Input: part model. Units: mm. Frame: model coordinates. Face numbers are marked on the shaded views. Coordinates: 2 decimals unless noted, no trailing zeros. Write each loop counter-clockwise with the first axis right and the second up, starting at its lowest first coordinate (ties: lowest second). Pieces come first, ordered by that corner, then holes.
1) Section query D-D (x = 42.5). Output: boundary loops of the cut face in (y, z), then the cut area to 3 significant figures.
2) Pin query (flat end, axial travel): pin 1 Ø4 at (x, y) = (44.5, 4) entering from +Z; pin 2 Ø5 at (x, z) = (67, -22) entering from +Y; pin 3 Ø16 at (x, z) = (38.09, -19.05) entering from +Y. Return the tip coordinate at first contact, or that it passes through.
3) Draft query along X for the marked faces 1, 2, 3 and 4. Return one class per face: pulls with the +X half, pulls with the -X half, needs draft (parallel to the pull), parting line crosses it, or undercut.
4) Section query B-B (y = 15). Output: boundary loops of the cut face in (x, z) (3 decimals), then the cut area to 3 significant figures.
5) Line query: L1, parallel to X at y = 8, z = -12.5; L2, parallel to Y at x = 38, z = -1.5; L3, parallel to X at y = 1.5, z = -19.05. Output: solid intervals per line, ascending.
6) Section query A-A (z = -19.05). Output: boundary loops of the cut face in (x, y), then the cut area to 3 significant figures.
7) Section query C-C (z = -3.5). Output: boundary loops of the cut face in (x, y), then the cut area to 3 significant figures.
from build123d import *

# Parameters (mm, degrees)
SKETCH1_W           = 76.2
SKETCH1_H           = 38.1
BOSS_EXTRUDE1_DEPTH = 25.4
SKETCH2_R           = 11.43
CUT_EXTRUDE1_DEPTH  = 89.9
SKETCH5_W           = 25.4
SKETCH5_H           = 5.08
CUT_EXTRUDE3_DEPTH  = 89.890839867
SKETCH3_R           = 3.302
CUT_EXTRUDE6_DEPTH  = 89.890839867
CUT_EXTRUDE7_START  = -7.62
SKETCH3_3_R         = 6.985
SKETCH3_3_R_2       = 3.302
CUT_EXTRUDE7_DEPTH  = 10.16


with BuildPart() as part:
    # Sketch1 → Boss-Extrude1 (new body)
    with BuildSketch(Plane(origin=(0, 0, 0), x_dir=(1, 0, 0), z_dir=(0, 1, 0))):
        with Locations((38.089312979, 19.05)):
            Rectangle(SKETCH1_W, SKETCH1_H)
    extrude(amount=BOSS_EXTRUDE1_DEPTH)

    # Sketch2 → Cut-Extrude1 (cut, through all)
    with BuildSketch(Plane.ZY.offset(0.010687021)):
        with Locations((-19.05, 25.4)):
            Circle(SKETCH2_R)
    extrude(amount=-CUT_EXTRUDE1_DEPTH, mode=Mode.SUBTRACT)

    # Sketch5 → Cut-Extrude3 (cut, through all)
    with BuildSketch(Plane(origin=(0, 0, -38.1), x_dir=(-1, 0, 0), z_dir=(0, 0, -1))):
        with Locations((-35.549312979, 8.89)):
            Rectangle(SKETCH5_W, SKETCH5_H)
    extrude(amount=-CUT_EXTRUDE3_DEPTH, mode=Mode.SUBTRACT)

    # Sketch3 → Cut-Extrude6 (cut, through all)
    with BuildSketch(Plane.XZ):
        with Locations(Location((38.089312979, -19.05, 0), (0, 0, 270))):
            Circle(SKETCH3_R)
    extrude(amount=-CUT_EXTRUDE6_DEPTH, mode=Mode.SUBTRACT)

    # Sketch3_3 → Cut-Extrude7 (cut)
    with BuildSketch(Plane.XZ.offset(CUT_EXTRUDE7_START)):
        with Locations(Location((38.089312979, -19.05, 0), (0, 0, 90))):
            Circle(SKETCH3_3_R)
        with Locations(Location((38.089312979, -19.05, 0), (0, 0, 270))):
            Circle(SKETCH3_3_R_2, mode=Mode.SUBTRACT)
    extrude(amount=-CUT_EXTRUDE7_DEPTH, mode=Mode.SUBTRACT)


solid = part.part
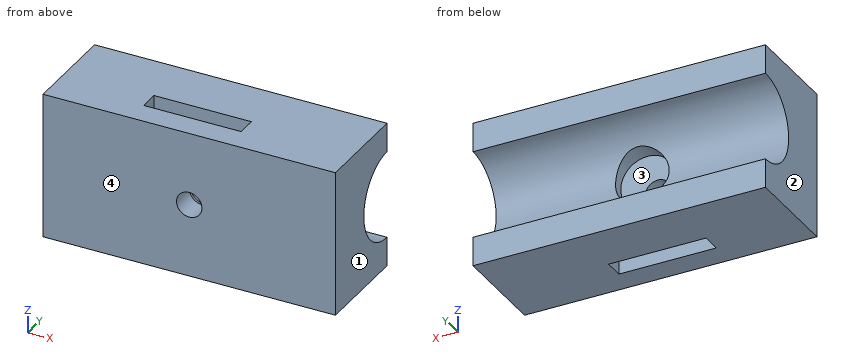
Answer:
1. outline: (0, -38.1) - (6.35, -38.1) - (6.35, 0) - (0, 0) - close; (11.43, -38.1) - (25.4, -38.1) - (25.4, -30.48) arc R11.43 cw to (15.33, -24.47) - (11.43, -24.47) - close; (11.43, -13.63) - (15.33, -13.63) arc R11.43 cw to (25.4, -7.62) - (25.4, 0) - (11.43, 0) - close
1. area: 537 mm2
2. pin 1: stops at z = 0
2. pin 2: stops at y = 15.35
2. pin 3: stops at y = 17.24
3. face 1: pulls with the +X half
3. face 2: pulls with the -X half
3. face 3: undercut
3. face 4: needs draft
4. outline: (-0.011, -38.1) - (76.189, -38.1) - (76.189, -23.792) - (43.218, -23.792) arc R6.985 cw to (32.96, -23.792) - (-0.011, -23.792) - close; (-0.011, -14.308) - (32.96, -14.308) arc R6.985 cw to (43.218, -14.308) - (76.189, -14.308) - (76.189, 0) - (-0.011, 0) - close
4. area: 2,150 mm2
5. L1: x = -0.01 to 22.85, 48.25 to 76.19
5. L2: y = 0 to 6.35, 11.43 to 25.4
5. L3: x = -0.01 to 34.79, 41.39 to 76.19
6. outline: (-0.01, 0) - (34.79, 0) - (34.79, 6.35) - (22.85, 6.35) - (22.85, 11.43) - (31.1, 11.43) - (31.1, 13.97) - (-0.01, 13.97) - close; (41.39, 0) - (76.19, 0) - (76.19, 13.97) - (45.07, 13.97) - (45.07, 11.43) - (48.25, 11.43) - (48.25, 6.35) - (41.39, 6.35) - close
6. area: 858 mm2
7. outline: (-0.01, 0) - (76.19, 0) - (76.19, 25.4) - (-0.01, 25.4) - close; hole (22.85, 6.35) - (48.25, 6.35) - (48.25, 11.43) - (22.85, 11.43) - close
7. area: 1,810 mm2
